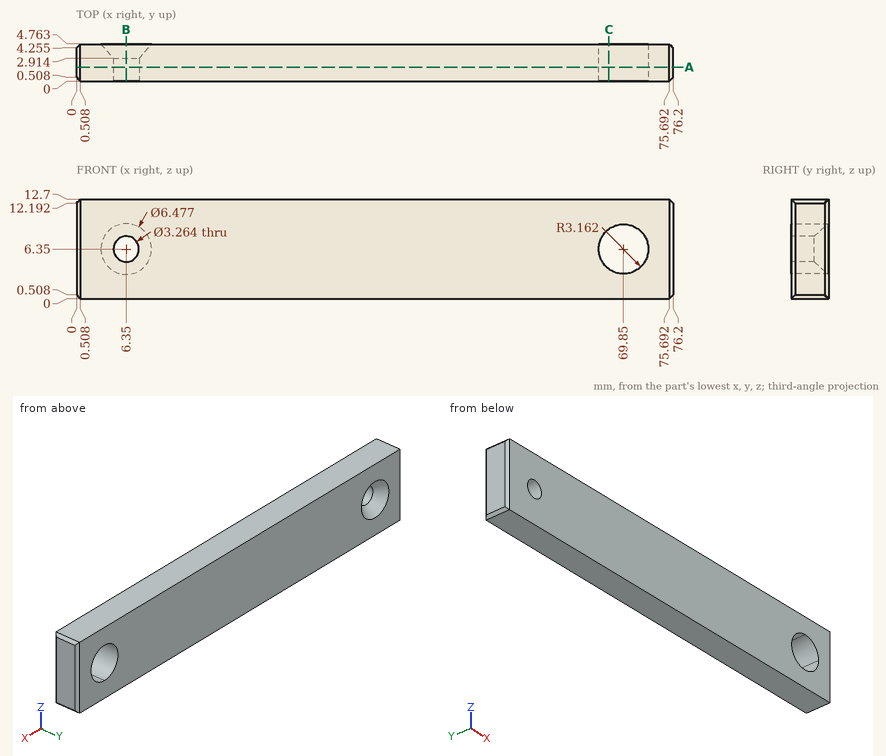
Design review of the part shown in the three views and the two pictorial views. Dimensions are in mm from the part's minimum x, y and z. Coordinates: 2 decimals unless noted, no trailing zeros. Write each loop counter-clockwise with the first axis right and the second up, starting at its lowest first coordinate (ties: lowest second). Pieces come first, ordered by that corner, then holes.
1) We need section C-C on x = 68. State the section outline as (y, z) points (1 decimal).
2) To check wall thickness, follow probe 1 along Z at (x, y) = (6.35, 2.2); probe 2 along X at (y, z) = (2.8, 6.75); probe 3 along X at (y, z) = (4.4, 6.75) (1 decimal). State the ranges of each line that lie inside material, in increasing order.
3) We need section A-A on y = 1.8. Count the separate pieces of the cut face and the enclosed holes in it.
4) We need section B-B on x = 6.35. State the section outline as (y, z) points (1 decimal).
Answer list:
1. outline: (0, 0) - (4.8, 0) - (4.8, 3.8) - (0, 3.8) - close; (0, 8.9) - (4.8, 8.9) - (4.8, 12.7) - (0, 12.7) - close
2. probe 1: z = 0 to 4.72, 7.98 to 12.7
2. probe 2: x = 0 to 4.77, 7.93 to 66.71, 72.99 to 76.2
2. probe 3: x = 0.1 to 3.5, 9.2 to 66.7, 73 to 76.1
3. separate pieces: 1
3. enclosed holes: 2
4. outline: (0, 0) - (4.8, 0) - (4.8, 3.1) - (2.9, 4.7) - (0, 4.7) - close; (0, 8) - (2.9, 8) - (4.8, 9.6) - (4.8, 12.7) - (0, 12.7) - close
